Geometry: final body of the model. Coordinates: model frame, mm. Face numbers are marked on the shaded views. Coordinates: 2 decimals unless noted, no trailing zeros. Write each loop counter-clockwise with the first axis right and the second up, starting at its lowest first coordinate (ties: lowest second). Pieces come first, ordered by that corner, then holes. Notation, with made-up numbers: (43.5, 5) -> (90.5, 5) arc R19 cw to (90.5, 29) -> close; hole circle Ø8 at (17.25, 48.5). An arc over 180 degrees is marked (long way). Answer as a JSON object with one key per item and string values. Group by question number.
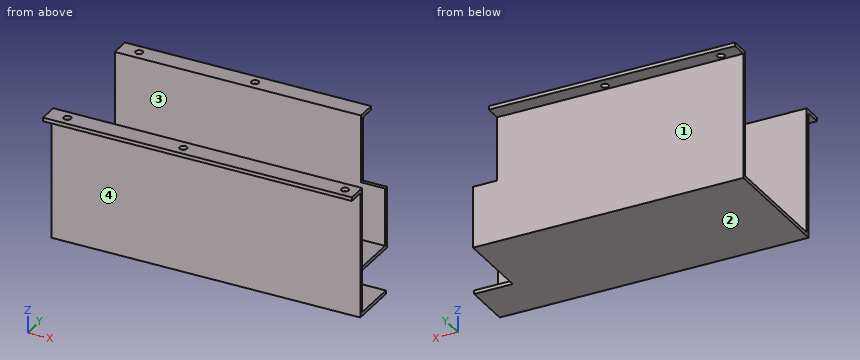
```python
from build123d import *

# Parameters (mm, degrees)
F1_DEPTH = 203.2
F2_W     = 82.55
F2_H     = 88.9
F3_DEPTH = 101.601
F4_W     = 50.8
F4_H     = 98.3996
F5_DEPTH = 169.8508
F6_R     = 4.7625
F7_DEPTH = 169.8508


with BuildPart() as f1:
    # F0 (on Right) → F1 (new body, symmetric)
    with BuildSketch(Plane.YZ):
        Polygon((76.2, 0), (-76.2, 0), (-76.2, 165.1), (-101.6, 165.1), (-101.6, 160.3502), (-80.9498, 160.3502), (-80.9498, -4.7498), (80.9498, -4.7498), (80.9498, 160.3502), (101.6, 160.3502), (101.6, 165.1), (76.2, 165.1), align=None)
    extrude(amount=F1_DEPTH, both=True)

    # F2 (on Front) → F3 (cut, through all)
    with BuildSketch(Plane.XZ):
        with Locations((161.925, 120.65)):
            Rectangle(F2_W, F2_H)
    extrude(amount=-F3_DEPTH, mode=Mode.SUBTRACT)

    # F4 (on face) → F5 (cut, through all)
    with BuildSketch(Plane(origin=(0, 0, -4.7498), x_dir=(1, 0, 0), z_dir=(0, 0, -1))):
        with Locations((177.8, -31.75)):
            Rectangle(F4_W, F4_H)
    extrude(amount=-F5_DEPTH, mode=Mode.SUBTRACT)

    # F6 (on face) → F7 (cut, through all)
    with BuildSketch(Plane.XY.offset(165.1)):
        with Locations((-177.8, 88.9)):
            Circle(F6_R)
        with Locations((-25.4, 88.9)):
            Circle(F6_R)
        with Locations((-177.8, -88.9)):
            Circle(F6_R)
        with Locations((-25.4, -88.9)):
            Circle(F6_R)
        with Locations((187.325, -88.9)):
            Circle(F6_R)
    extrude(amount=-F7_DEPTH, mode=Mode.SUBTRACT)


solid = f1.part
```
Item 1: Section D-D on x = -25.4. Output: boundary loops of the cut face in (y, z).
Item 2: Section B-B on z = 21.5. Output: boundary loops of the cut face in (x, y).
Item 3: Section C-C on y = 88.9. Output: boundary loops of the cut face in (x, z).
Item 4: Section A-A on y = -88.9. Output: boundary loops of the cut face in (x, z), then the cut area to 3 significant figures.
Item 5: Mould query, pull axis Y, two halves, no side actions, for the marked faces 1, 2, 3 and 4. Classes: +Y half, -Y half, draft (parallel to the pull), parting line (faces both ways), or undercut.
Item 6: Ray query, L1, parallel to Y at x = -177, z = 163; L2, parallel to Y at x = -144.5, z = 23; L3, parallel to Y at x = -177.8, z = 161.9. Return the intervals inside material, ascending. Write a range as [from, to].
Item 7: Contact query for flat-ended pins moving along their axis: pin 1 (7.5 mm diameter, centred on x = -25.4, y = -88.9, fed in from +Z); pin 2 (3 mm diameter, centred on x = -16, y = 72.5, fed in from +Z); pin 3 (1.4 mm diameter, centred on x = 133.5, y = 79, fed in from +Z); pin 4 (15 mm diameter, centred on x = -25.4, y = 88.9, fed in from -Z). Output: stop coordinate, or through.
Answer sheet:
{
 "1": {"outline": "(-101.6, 160.35) -> (-93.66, 160.35) -> (-93.66, 165.1) -> (-101.6, 165.1) -> close; (-84.14, 160.35) -> (-80.95, 160.35) -> (-80.95, -4.75) -> (80.95, -4.75) -> (80.95, 160.35) -> (84.14, 160.35) -> (84.14, 165.1) -> (76.2, 165.1) -> (76.2, 0) -> (-76.2, 0) -> (-76.2, 165.1) -> (-84.14, 165.1) -> close; (93.66, 160.35) -> (101.6, 160.35) -> (101.6, 165.1) -> (93.66, 165.1) -> close"},
 "2": {"outline": "(-203.2, -80.95) -> (203.2, -80.95) -> (203.2, -76.2) -> (-203.2, -76.2) -> close; (-203.2, 76.2) -> (152.4, 76.2) -> (152.4, 80.95) -> (-203.2, 80.95) -> close"},
 "3": {"outline": "(-203.2, 160.35) -> (-182.56, 160.35) -> (-182.56, 165.1) -> (-203.2, 165.1) -> close; (-173.04, 160.35) -> (-30.16, 160.35) -> (-30.16, 165.1) -> (-173.04, 165.1) -> close; (-20.64, 160.35) -> (120.65, 160.35) -> (120.65, 165.1) -> (-20.64, 165.1) -> close"},
 "4": {"outline": "(-203.2, 160.35) -> (-182.56, 160.35) -> (-182.56, 165.1) -> (-203.2, 165.1) -> close; (-173.04, 160.35) -> (-30.16, 160.35) -> (-30.16, 165.1) -> (-173.04, 165.1) -> close; (-20.64, 160.35) -> (182.56, 160.35) -> (182.56, 165.1) -> (-20.64, 165.1) -> close; (192.09, 160.35) -> (203.2, 160.35) -> (203.2, 165.1) -> (192.09, 165.1) -> close", "area": "1,790 mm^2"},
 "5": {"face 1": "+Y half", "face 2": "draft", "face 3": "undercut", "face 4": "-Y half"},
 "6": {"L1": "y = [-101.6, -93.59], [-84.21, -76.2], [76.2, 84.21], [93.59, 101.6]", "L2": "y = [-80.95, -76.2], [76.2, 80.95]", "L3": "y = [-101.6, -93.66], [-84.14, -76.2], [76.2, 84.14], [93.66, 101.6]"},
 "7": {"pin 1": "passes through", "pin 2": "stops at z = 0", "pin 3": "stops at z = 76.2", "pin 4": "stops at z = 160.35"}
}
